The model under review builds one solid part; all positions refer to its coordinate system, in mm. Round coordinates to 2 decimals unless told otherwise and drop trailing zeros. Order: outer loops, then holes, each group sorted by start corner. A loop starts at its lowest first (then second) coordinate and runs counter-clockwise, first axis right, second up.
1) Mouldability with a two-part tool opening along Y and no side actions: class faces 1 (the face through (2, 10, 0)), 2 (the face through (1.713, 29.222, 57.923)), 3 (the face through (2, 49.591, 40)) as pulls with the +Y half, pulls with the -Y half, needs draft (parallel to the pull), parting line crosses it, or undercut.
2) Consider section A-A (x = -17). Give the boundary of the cut face in (y, z), then the cut area to 3 significant figures.
3) To check wall thickness, follow L1, parallel to Y at x = -6.5, z = 46; L2, parallel to Z at x = -16.5, y = 16.5; L3, parallel to Y at x = 37, z = 45.5. State the ranges of each line that lie inside material, in increasing order.
from build123d import *

# Parameters (mm, degrees)
F0_W     = 80
F0_H     = 80
F1_DEPTH = 80
F2_R     = 17.08616193
F3_DEPTH = 80.001
F4_R     = 5


with BuildPart() as f1:
    # F0 (on Top) → F1 (new body)
    with BuildSketch(Plane.XY):
        with Locations((2.2027976811, 9.5911924709)):
            Rectangle(F0_W, F0_H)
    extrude(amount=F1_DEPTH)

    # F2 (on face) → F3 (cut, through all)
    with BuildSketch(Plane(origin=(-37.7972023189, 0, 0), x_dir=(0, -1, 0), z_dir=(-1, 0, 0))):
        with Locations((-16.629083944, 46.3755141786)):
            Circle(F2_R)
    extrude(amount=-F3_DEPTH, mode=Mode.SUBTRACT)

    # F4
    f4_edges = [f1.edges().sort_by_distance(p)[0] for p in [
        (-37.797202, 49.591192, 40),
        (-37.797202, 9.591192, 80),
        (-37.797202, -30.408808, 40),
        (-37.797202, 9.591192, 0),
        (-37.797202, 33.715246, 46.375514),
        (42.202798, 49.591192, 40),
        (2.202798, 49.591192, 0),
        (2.202798, 49.591192, 80),
        (42.202798, -30.408808, 40),
        (42.202798, 9.591192, 80),
        (42.202798, 9.591192, 0),
        (42.202798, 33.715246, 46.375514),
        (2.202798, -30.408808, 0),
        (2.202798, -30.408808, 80),
    ]]
    fillet(f4_edges, radius=F4_R)


solid = f1.part
Answer below:
1. face 1: needs draft
1. face 2: undercut
1. face 3: pulls with the +Y half
2. outline: (-30.41, 5) arc R5 ccw to (-25.41, 0) - (44.59, 0) arc R5 ccw to (49.59, 5) - (49.59, 75) arc R5 ccw to (44.59, 80) - (-25.41, 80) arc R5 ccw to (-30.41, 75) - close; hole circle Ø34.17 at (16.63, 46.38)
2. area: 5,460 mm2
3. L1: y = -30.41 to -0.45, 33.71 to 49.59
3. L2: z = 0 to 29.29, 63.46 to 80
3. L3: y = -30.41 to -0.43, 33.69 to 49.59
